Read the model definition and answer for the solid it produces. Units are mm, in the model's axes. Face numbers are marked on the shaded views. Coordinates: 2 decimals unless noted, no trailing zeros. Write each loop counter-clockwise with the first axis right and the second up, starting at its lowest first coordinate (ties: lowest second). Pieces come first, ordered by that corner, then holes. Notation, with made-up numbers: (48.5, 25) -> (103.5, 25) arc R28 cw to (103.5, 62) -> close; hole circle Ø8 at (-8, 45). An arc over 180 degrees is marked (long way). Use CSV: the item, a comma, the result in double quotes.
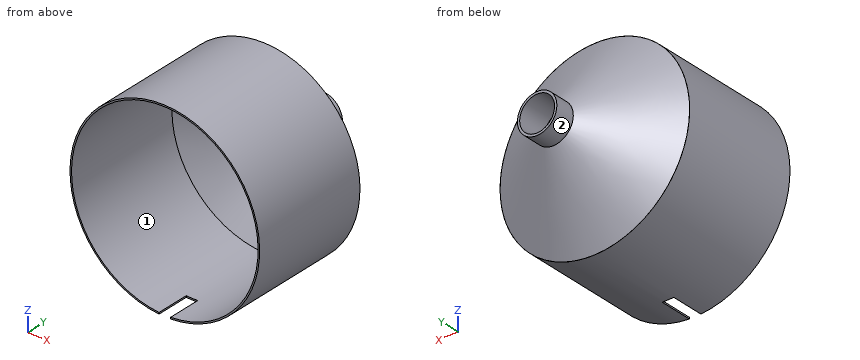
from build123d import *

# Parameters (mm, degrees)
SKETCH1_R           = 62.5
SKETCH1_R_2         = 61.5
BOSS_EXTRUDE1_DEPTH = 80
SKETCH3_W           = 7.6
SKETCH3_H           = 23.660429452
CUT_EXTRUDE1_DEPTH  = 80
SKETCH5_R           = 12.3
CUT_EXTRUDE3_DEPTH  = 229
BOSS_EXTRUDE3_START = 106
SKETCH6_R           = 13
SKETCH6_R_2         = 11.5
BOSS_EXTRUDE3_DEPTH = 20


with BuildPart() as part:
    # Sketch1 → Boss-Extrude1 (new body)
    with BuildSketch(Plane(origin=(0, 0, 0), x_dir=(1, 0, 0), z_dir=(0, 1, 0))):
        with Locations(Location((0, 0, 0), (0, 0, 270))):
            Circle(SKETCH1_R)
        with Locations(Location((0, 0, 0), (0, 0, 270))):
            Circle(SKETCH1_R_2, mode=Mode.SUBTRACT)
    extrude(amount=BOSS_EXTRUDE1_DEPTH)

    # Sketch2 → Revolve1 (revolve)
    with BuildSketch(Plane.XY, mode=Mode.PRIVATE) as revolve1_sk:
        Polygon((-62.472592019, 80), (-62.472592019, 79.276884175), (-61.5, 79.276884175), (-61.5, 80), (-4.8, 117.682815259), (-4.8, 129.995512562), (-8, 129.995512562), (-8, 127), (-6.8, 127), (-6.8, 117), align=None)
    revolve(revolve1_sk.sketch.rotate(Axis((0, 80, 0), (0, 1, 0)), 270), axis=Axis((0, 80, 0), (0, 1, 0)))

    # Sketch3 → Cut-Extrude1 (cut)
    with BuildSketch(Plane.XY):
        with Locations((0, 9.876009184)):
            Rectangle(SKETCH3_W, SKETCH3_H)
    extrude(amount=-CUT_EXTRUDE1_DEPTH, mode=Mode.SUBTRACT)

    # Sketch5 → Cut-Extrude3 (cut)
    with BuildSketch(Plane(origin=(0, 0, 0), x_dir=(1, 0, 0), z_dir=(0, 1, 0))):
        with Locations(Location((0, 0, 0), (0, 0, 90))):
            Circle(SKETCH5_R)
    extrude(amount=CUT_EXTRUDE3_DEPTH, mode=Mode.SUBTRACT)

    # Sketch6 → Boss-Extrude3 (add)
    with BuildSketch(Plane(origin=(0, 0, 0), x_dir=(1, 0, 0), z_dir=(0, 1, 0)).offset(BOSS_EXTRUDE3_START)):
        with Locations(Location((0, 0, 0), (0, 0, 90))):
            Circle(SKETCH6_R)
        with Locations(Location((0, 0, 0), (0, 0, 270))):
            Circle(SKETCH6_R_2, mode=Mode.SUBTRACT)
    extrude(amount=BOSS_EXTRUDE3_DEPTH)


solid = part.part
1. A cutting plane is placed at D-D (y = 115). Give the vertices of the cut face in (x, z), and give its area (3 significant figures).
Solutions:
outline,"circle Ø26 at (0, 0); hole circle Ø23 at (0, 0)"
area,"115 mm^2"
2. A cutting plane is placed at C-C (y = 38). Give the vertices of the cut face in (x, z), and give its area (3 significant figures).
Solutions:
outline,"circle Ø125 at (0, 0); hole circle Ø123 at (0, 0)"
area,"390 mm^2"
3. For a pull along X with two mould halves and no side action, classify the marked faces 1 and 2 as pulls with the +X half, pulls with the -X half, needs draft (parallel to the pull), parting line crosses it, or undercut.
Solutions:
face 1,"undercut"
face 2,"parting line crosses it"
4. Each of these flat-tipped pins is pushed along its axis until it touches: pin 1 Ø2 at (y, z) = (99.5, -12) entering from +X; pin 2 Ø3 at (x, y) = (31.5, 102.5) entering from -Z; pin 3 Ø0.6 at (x, z) = (2, -62) entering from -Y; pin 4 Ø10 at (y, z) = (27, -48) entering from +X. Where does it stop, or does it pass through?
Solutions:
pin 1,"stops at x = 32.53"
pin 2,"passes through"
pin 3,"stops at y = 21.71"
pin 4,"stops at x = 45.36"
5. Find the intervals of material crossed by line 1 along Z through (x, y) = (0, 33.5); line 2 along X through (y, z) = (113, 0), in increasing order.
Solutions:
line 1,"z = -62.5 to -61.5, 61.5 to 62.5"
line 2,"x = -13 to -11.5, 11.5 to 13"
